Build history of the part. All positions in model axes, mm. A direction names the side the tool comes from. Give positions to 0.01 mm unless a question says otherwise; leave off trailing zeros. Loops run counter-clockwise (first coordinate to the right, second up) from the corner with the lowest first, then second, coordinate; pieces in that order, holes last. Notation, with made-up numbers: M 20.5,29.25 L 28.5,29.25 A11 ccw 28.5,33.25 Z; hole C -4.5,60 d8. An arc over 180 degrees is marked long. Put each result on its own line as item: value.
```python
from build123d import *

# Parameters (mm, degrees)
F0_R     = 12
F1_DEPTH = 4
F2_DEPTH = 4


# Not quite as in the source:
# - a feature names something its author has since deleted; it is built from what else it names


with BuildPart() as f1:
    # F0 (on Top) → F1 (new body)
    with BuildSketch(Plane.XY):
        with BuildLine():
            Line((64.1499952853, -10.0000936452), (64.1499952853, 9.9999063548))
            ThreePointArc((64.1499952853, 9.9999063548), (56.8276648149, 27.6775758844), (39.1499952853, 34.9999063548))
            Line((39.1499952853, 34.9999063548), (-48.3500047147, 29.9999063548))
            ThreePointArc((-48.3500047147, 29.9999063548), (-78.3500047147, -9.36452e-05), (-48.3500047147, -30.0000936452))
            Line((-48.3500047147, -30.0000936452), (39.1499952853, -35.0000936452))
            ThreePointArc((39.1499952853, -35.0000936452), (56.8276648149, -27.6777631749), (64.1499952853, -10.0000936452))
        make_face()
        with BuildLine():
            ThreePointArc((-0.5500047147, -19.1500936452), (-4.4500047147, -15.2500936452), (-0.5500047147, -11.3500936452))
            Line((-0.5500047147, -11.3500936452), (24.1499952853, -11.3500936452))
            Line((24.1499952853, -11.3500936452), (48.8499952853, -11.3500936452))
            ThreePointArc((48.8499952853, -11.3500936452), (52.7499952853, -15.2500936452), (48.8499952853, -19.1500936452))
            Line((48.8499952853, -19.1500936452), (24.1499952853, -19.1500936452))
            Line((24.1499952853, -19.1500936452), (-0.5500047147, -19.1500936452))
        make_face(mode=Mode.SUBTRACT)
        with Locations((-48.3500047147, -9.36452e-05)):
            Circle(F0_R, mode=Mode.SUBTRACT)
        with BuildLine():
            ThreePointArc((-55.1419234399, 14.5971608922), (-61.784523832, 17.0211782252), (-59.3605064989, 23.6637786173))
            ThreePointArc((-59.3605064989, 23.6637786173), (-50.6247696004, 26.0005879749), (-41.615965488, 25.2162247953))
            ThreePointArc((-41.615965488, 25.2162247953), (-38.075298972, 19.0954666215), (-44.1960571458, 15.5548001054))
            ThreePointArc((-44.1960571458, 15.5548001054), (-49.753212173, 16.038640994), (-55.1419234399, 14.5971608922))
        make_face(mode=Mode.SUBTRACT)
        with BuildLine():
            Line((24.1499952853, 5.9999063548), (32.6499952853, 5.9999063548))
            ThreePointArc((32.6499952853, 5.9999063548), (38.6499952853, -9.36452e-05), (32.6499952853, -6.0000936452))
            Line((32.6499952853, -6.0000936452), (24.1499952853, -6.0000936452))
            Line((24.1499952853, -6.0000936452), (15.6499952853, -6.0000936452))
            ThreePointArc((15.6499952853, -6.0000936452), (9.6499952853, -9.36452e-05), (15.6499952853, 5.9999063548))
            Line((15.6499952853, 5.9999063548), (24.1499952853, 5.9999063548))
        make_face(mode=Mode.SUBTRACT)
        with BuildLine():
            Line((24.1499952853, 11.3499063548), (-0.5500047147, 11.3499063548))
            ThreePointArc((-0.5500047147, 11.3499063548), (-4.4500047147, 15.2499063548), (-0.5500047147, 19.1499063548))
            Line((-0.5500047147, 19.1499063548), (24.1499952853, 19.1499063548))
            Line((24.1499952853, 19.1499063548), (48.8499952853, 19.1499063548))
            ThreePointArc((48.8499952853, 19.1499063548), (52.7499952853, 15.2499063548), (48.8499952853, 11.3499063548))
            Line((48.8499952853, 11.3499063548), (24.1499952853, 11.3499063548))
        make_face(mode=Mode.SUBTRACT)
        with BuildLine():
            ThreePointArc((-41.615965488, 25.2162247953), (-50.6247696004, 26.0005879749), (-59.3605064989, 23.6637786173))
            ThreePointArc((-59.3605064989, 23.6637786173), (-61.784523832, 17.0211782252), (-55.1419234399, 14.5971608922))
            ThreePointArc((-55.1419234399, 14.5971608922), (-49.753212173, 16.038640994), (-44.1960571458, 15.5548001054))
            ThreePointArc((-44.1960571458, 15.5548001054), (-38.075298972, 19.0954666215), (-41.615965488, 25.2162247953))
        make_face()
        with BuildLine():
            ThreePointArc((-56.0278258823, 16.5011506145), (-59.8805341097, 17.9070806676), (-58.4746040565, 21.7597888951))
            ThreePointArc((-58.4746040565, 21.7597888951), (-50.4417425407, 23.908579109), (-42.1577847361, 23.1873256104))
            ThreePointArc((-42.1577847361, 23.1873256104), (-40.1041981568, 19.6372858696), (-43.6542378976, 17.5836992903))
            ThreePointArc((-43.6542378976, 17.5836992903), (-49.9362392327, 18.13064986), (-56.0278258823, 16.5011506145))
        make_face(mode=Mode.SUBTRACT)
        with BuildLine():
            ThreePointArc((-0.5500047147, 19.1499063548), (-4.4500047147, 15.2499063548), (-0.5500047147, 11.3499063548))
            Line((-0.5500047147, 11.3499063548), (24.1499952853, 11.3499063548))
            Line((24.1499952853, 11.3499063548), (48.8499952853, 11.3499063548))
            ThreePointArc((48.8499952853, 11.3499063548), (52.7499952853, 15.2499063548), (48.8499952853, 19.1499063548))
            Line((48.8499952853, 19.1499063548), (24.1499952853, 19.1499063548))
            Line((24.1499952853, 19.1499063548), (-0.5500047147, 19.1499063548))
        make_face()
        with BuildLine():
            Line((24.1499952853, 13.0499063548), (-0.5500047147, 13.0499063548))
            ThreePointArc((-0.5500047147, 13.0499063548), (-2.7500047147, 15.2499063548), (-0.5500047147, 17.4499063548))
            Line((-0.5500047147, 17.4499063548), (24.1499952853, 17.4499063548))
            Line((24.1499952853, 17.4499063548), (48.8499952853, 17.4499063548))
            ThreePointArc((48.8499952853, 17.4499063548), (51.0499952853, 15.2499063548), (48.8499952853, 13.0499063548))
            Line((48.8499952853, 13.0499063548), (24.1499952853, 13.0499063548))
        make_face(mode=Mode.SUBTRACT)
        with BuildLine():
            Line((24.1499952853, -11.3500936452), (-0.5500047147, -11.3500936452))
            ThreePointArc((-0.5500047147, -11.3500936452), (-4.4500047147, -15.2500936452), (-0.5500047147, -19.1500936452))
            Line((-0.5500047147, -19.1500936452), (24.1499952853, -19.1500936452))
            Line((24.1499952853, -19.1500936452), (48.8499952853, -19.1500936452))
            ThreePointArc((48.8499952853, -19.1500936452), (52.7499952853, -15.2500936452), (48.8499952853, -11.3500936452))
            Line((48.8499952853, -11.3500936452), (24.1499952853, -11.3500936452))
        make_face()
        with BuildLine():
            ThreePointArc((-0.5500047147, -17.4500936452), (-2.7500047147, -15.2500936452), (-0.5500047147, -13.0500936452))
            Line((-0.5500047147, -13.0500936452), (24.1499952853, -13.0500936452))
            Line((24.1499952853, -13.0500936452), (48.8499952853, -13.0500936452))
            ThreePointArc((48.8499952853, -13.0500936452), (51.0499952853, -15.2500936452), (48.8499952853, -17.4500936452))
            Line((48.8499952853, -17.4500936452), (24.1499952853, -17.4500936452))
            Line((24.1499952853, -17.4500936452), (-0.5500047147, -17.4500936452))
        make_face(mode=Mode.SUBTRACT)
    extrude(amount=-F1_DEPTH)

    # F0 (on Top) → F2 (join)
    with BuildSketch(Plane.XY):
        with BuildLine():
            Line((64.1499952853, -10.0000936452), (64.1499952853, 9.9999063548))
            ThreePointArc((64.1499952853, 9.9999063548), (56.8276648149, 27.6775758844), (39.1499952853, 34.9999063548))
            Line((39.1499952853, 34.9999063548), (-48.3500047147, 29.9999063548))
            ThreePointArc((-48.3500047147, 29.9999063548), (-78.3500047147, -9.36452e-05), (-48.3500047147, -30.0000936452))
            Line((-48.3500047147, -30.0000936452), (39.1499952853, -35.0000936452))
            ThreePointArc((39.1499952853, -35.0000936452), (56.8276648149, -27.6777631749), (64.1499952853, -10.0000936452))
        make_face()
        with BuildLine():
            ThreePointArc((-0.5500047147, -19.1500936452), (-4.4500047147, -15.2500936452), (-0.5500047147, -11.3500936452))
            Line((-0.5500047147, -11.3500936452), (24.1499952853, -11.3500936452))
            Line((24.1499952853, -11.3500936452), (48.8499952853, -11.3500936452))
            ThreePointArc((48.8499952853, -11.3500936452), (52.7499952853, -15.2500936452), (48.8499952853, -19.1500936452))
            Line((48.8499952853, -19.1500936452), (24.1499952853, -19.1500936452))
            Line((24.1499952853, -19.1500936452), (-0.5500047147, -19.1500936452))
        make_face(mode=Mode.SUBTRACT)
        with Locations((-48.3500047147, -9.36452e-05)):
            Circle(F0_R, mode=Mode.SUBTRACT)
        with BuildLine():
            ThreePointArc((-55.1419234399, 14.5971608922), (-61.784523832, 17.0211782252), (-59.3605064989, 23.6637786173))
            ThreePointArc((-59.3605064989, 23.6637786173), (-50.6247696004, 26.0005879749), (-41.615965488, 25.2162247953))
            ThreePointArc((-41.615965488, 25.2162247953), (-38.075298972, 19.0954666215), (-44.1960571458, 15.5548001054))
            ThreePointArc((-44.1960571458, 15.5548001054), (-49.753212173, 16.038640994), (-55.1419234399, 14.5971608922))
        make_face(mode=Mode.SUBTRACT)
        with BuildLine():
            Line((24.1499952853, 5.9999063548), (32.6499952853, 5.9999063548))
            ThreePointArc((32.6499952853, 5.9999063548), (38.6499952853, -9.36452e-05), (32.6499952853, -6.0000936452))
            Line((32.6499952853, -6.0000936452), (24.1499952853, -6.0000936452))
            Line((24.1499952853, -6.0000936452), (15.6499952853, -6.0000936452))
            ThreePointArc((15.6499952853, -6.0000936452), (9.6499952853, -9.36452e-05), (15.6499952853, 5.9999063548))
            Line((15.6499952853, 5.9999063548), (24.1499952853, 5.9999063548))
        make_face(mode=Mode.SUBTRACT)
        with BuildLine():
            Line((24.1499952853, 11.3499063548), (-0.5500047147, 11.3499063548))
            ThreePointArc((-0.5500047147, 11.3499063548), (-4.4500047147, 15.2499063548), (-0.5500047147, 19.1499063548))
            Line((-0.5500047147, 19.1499063548), (24.1499952853, 19.1499063548))
            Line((24.1499952853, 19.1499063548), (48.8499952853, 19.1499063548))
            ThreePointArc((48.8499952853, 19.1499063548), (52.7499952853, 15.2499063548), (48.8499952853, 11.3499063548))
            Line((48.8499952853, 11.3499063548), (24.1499952853, 11.3499063548))
        make_face(mode=Mode.SUBTRACT)
    extrude(amount=F2_DEPTH)


solid = f1.part
```
Q1. Probe line 1 (Y direction, x = 33, z = 2); line 2 (X direction, y = 17, z = 1.25); line 3 (Y direction, x = 20, z = 2.75). List the from-to ranges inside material, lowest first. Write a range as from..to.
Here are the results:
line 1: -34.65..-19.15, -11.35..-5.99, 5.99..11.35, 19.15..34.65
line 2: -73.07..-61.77, -39.23..-4.04, 52.34..63.15
line 3: -33.91..-19.15, -11.35..-6, 6..11.35, 19.15..33.91
Q2. Slice it at A-A (x = 19). List the corners of the cut face in (y, z).
Here are the results:
outline: M -33.85,-4 L -17.45,-4 L -17.45,0 L -19.15,0 L -19.15,4 L -33.85,4 Z; M -13.05,-4 L -6,-4 L -6,4 L -11.35,4 L -11.35,0 L -13.05,0 Z; M 6,-4 L 13.05,-4 L 13.05,0 L 11.35,0 L 11.35,4 L 6,4 Z; M 17.45,-4 L 33.85,-4 L 33.85,4 L 19.15,4 L 19.15,0 L 17.45,0 Z
Q3. Mould opens along Y. For faces 1 (the flat face through (-5.213, -32.465, -0.056)), 2 (the flat face through (8, 0, 4)), 3 (the flat face through (24, -19.15, 2)) say: pulls with the +Y half, pulls with the -Y half, needs draft (parallel to the pull), parting line crosses it, or undercut.
Here are the results:
face 1: pulls with the -Y half
face 2: needs draft
face 3: undercut
Q4. Slice it at B-B (x = -51.5). List the corners of the cut face in (y, z), and give its area (3 significant figures).
Here are the results:
outline: M -29.83,-4 L -11.58,-4 L -11.58,4 L -29.83,4 Z; M 11.58,-4 L 17.93,-4 L 17.93,0 L 15.79,0 L 15.79,4 L 11.58,4 Z; M 23.79,-4 L 29.83,-4 L 29.83,4 L 25.91,4 L 25.91,0 L 23.79,0 Z
area: 228 mm²
Q5. Slice it at D-D (y = -25). List the corners of the cut face in (x, z), and give its area (3 significant figures).
Here are the results:
outline: M -64.93,-4 L 59.15,-4 L 59.15,4 L -64.93,4 Z
area: 993 mm²
Q6. Tool access for faces 4 (the flat face through (24, 17.45, -2)), 5 (the cylindrical face through (56.6, -27.9, -0.1)), 6 (the cylindrical face through (52.75, -15.16, 1.97)): list every direction of +Z, -Z, +X, -X, +Y, -Y with a clear straight run to the whole face (end or side of a thin tool).
Here are the results:
face 4: +Z, -Z
face 5: +Z, -Z, +X, -Y
face 6: +Z
Q7. Drop flat-ended pins along their axis: pin 1 Ø2 at (x, z) = (15.5, 1.5) entering from -Y; pin 2 Ø2 at (x, z) = (13.5, -2.5) entering from +Y; pin 3 Ø2 at (x, z) = (-20.5, -2.5) entering from -Y. Give the stop position or say it passes through.
Here are the results:
pin 1: y = -33.71
pin 2: y = 33.59
pin 3: y = -31.65
Q8. Slice it at C-C (z = 2.5). List the corners of the cut face in (x, y).
Here are the results:
outline: M -48.35,-30 L 39.15,-35 A25 ccw 64.15,-10 L 64.15,10 A25 ccw 39.15,35 L -48.35,30 A30 ccw Z; hole C -48.35,0 d24; hole M -59.36,23.66 A5 ccw -55.14,14.6 A16.1 cw -44.2,15.55 A5 ccw -41.62,25.22 A26.1 ccw Z; hole M -0.55,-19.15 L 48.85,-19.15 A3.9 ccw 48.85,-11.35 L -0.55,-11.35 A3.9 ccw Z; hole M -0.55,11.35 L 48.85,11.35 A3.9 ccw 48.85,19.15 L -0.55,19.15 A3.9 ccw Z; hole M 15.65,-6 L 32.65,-6 A6 ccw 32.65,6 L 15.65,6 A6 ccw Z
